```python
from build123d import *

# Parameters (mm, degrees)
SKETCH1_R           = 1
BOSS_EXTRUDE1_DEPTH = 8
SKETCH2_R           = 7
SKETCH2_R_2         = 3
CUT_EXTRUDE1_DEPTH  = 4
SKETCH3_R           = 3
CUT_EXTRUDE2_DEPTH  = 1.5
SKETCH8_R           = 3
BOSS_EXTRUDE4_DEPTH = 3
SKETCH9_W           = 12
SKETCH9_H           = 7
CUT_EXTRUDE5_DEPTH  = 19
SKETCH10_R          = 4.5
CUT_EXTRUDE11_DEPTH = 5
SKETCH12_R          = 3
CUT_EXTRUDE12_DEPTH = 5
SKETCH13_W          = 28.183943327
SKETCH13_H          = 2
CUT_EXTRUDE13_DEPTH = 19
BOSS_EXTRUDE5_REACH = 20
SKETCH14_W          = 8.331719186
SKETCH14_H          = 2


with BuildPart() as part:
    # Sketch1 → Boss-Extrude1 (new body)
    with BuildSketch(Plane(origin=(0, 0, 0), x_dir=(1, 0, 0), z_dir=(0, 1, 0))):
        with BuildLine():
            Line((-3, 53.504881109), (15, 53.504881109))
            Line((15, 53.504881109), (15, 23.504881109))
            ThreePointArc((15, 23.504881109), (6, 14.504881109), (-3, 23.504881109))
            Line((-3, 23.504881109), (-3, 53.504881109))
        make_face()
        with Locations((6, 36.504881109)):
            Circle(SKETCH1_R, mode=Mode.SUBTRACT)
        with Locations((6, 46.504881109)):
            Circle(SKETCH1_R, mode=Mode.SUBTRACT)
    extrude(amount=BOSS_EXTRUDE1_DEPTH)

    # Sketch2 → Cut-Extrude1 (cut)
    with BuildSketch(Plane(origin=(0, 8, 0), x_dir=(1, 0, 0), z_dir=(0, 1, 0))):
        with Locations((6, 23.504881109)):
            Circle(SKETCH2_R)
        with Locations((6, 23.504881109)):
            Circle(SKETCH2_R_2, mode=Mode.SUBTRACT)
    extrude(amount=-CUT_EXTRUDE1_DEPTH, mode=Mode.SUBTRACT)

    # Sketch3 → Cut-Extrude2 (cut)
    with BuildSketch(Plane(origin=(0, 8, 0), x_dir=(1, 0, 0), z_dir=(0, 1, 0))):
        with Locations((6, 23.504881109)):
            Circle(SKETCH3_R)
    extrude(amount=-CUT_EXTRUDE2_DEPTH, mode=Mode.SUBTRACT)

    # Sketch8 → Boss-Extrude4 (add)
    with BuildSketch(Plane(origin=(0, 8, 0), x_dir=(1, 0, 0), z_dir=(0, 1, 0))):
        with BuildLine():
            Line((1, 39.504881109), (11, 39.504881109))
            Line((11, 39.504881109), (15, 39.504881109))
            Line((15, 39.504881109), (15, 46.504881109))
            ThreePointArc((15, 46.504881109), (6, 51.504881109), (-3, 46.504881109))
            Line((-3, 46.504881109), (-3, 39.504881109))
            Line((-3, 39.504881109), (1, 39.504881109))
        make_face()
        with Locations((6, 46.504881109)):
            Circle(SKETCH8_R, mode=Mode.SUBTRACT)
    extrude(amount=BOSS_EXTRUDE4_DEPTH)

    # Sketch9 → Cut-Extrude5 (cut, through all)
    with BuildSketch(Plane(origin=(15, 0, 0), x_dir=(0, 0, -1), z_dir=(1, 0, 0))):
        with Locations((47.504881109, 3.5)):
            Rectangle(SKETCH9_W, SKETCH9_H)
    extrude(amount=-CUT_EXTRUDE5_DEPTH, mode=Mode.SUBTRACT)

    # Sketch10 → Cut-Extrude11 (cut)
    with BuildSketch(Plane(origin=(0, 8, 0), x_dir=(1, 0, 0), z_dir=(0, 1, 0))):
        with Locations((6, 36.504881109)):
            Circle(SKETCH10_R)
    extrude(amount=CUT_EXTRUDE11_DEPTH, mode=Mode.SUBTRACT)

    # Sketch12 → Cut-Extrude12 (cut)
    with BuildSketch(Plane(origin=(0, 8, 0), x_dir=(1, 0, 0), z_dir=(0, 1, 0))):
        with Locations((6, 46.504881109)):
            Circle(SKETCH12_R)
        with BuildLine():
            Line((-3, 53.504881109), (15, 53.504881109))
            Line((15, 53.504881109), (15, 46.504881109))
            ThreePointArc((15, 46.504881109), (6, 51.504881109), (-3, 46.504881109))
            Line((-3, 46.504881109), (-3, 53.504881109))
        make_face()
    extrude(amount=-CUT_EXTRUDE12_DEPTH, mode=Mode.SUBTRACT)

    # Sketch13 → Cut-Extrude13 (cut, through all)
    with BuildSketch(Plane(origin=(15, 0, 0), x_dir=(0, 0, -1), z_dir=(1, 0, 0))):
        with Locations((27.412909446, 1)):
            Rectangle(SKETCH13_W, SKETCH13_H)
    extrude(amount=-CUT_EXTRUDE13_DEPTH, mode=Mode.SUBTRACT)

    # Sketch14 → Boss-Extrude5 (add, up to next)
    with BuildSketch(Plane(origin=(15, 0, 0), x_dir=(0, 0, -1), z_dir=(1, 0, 0)), mode=Mode.PRIVATE) as boss_extrude5_sk1:
        with Locations((37.339021516, 3)):
            Rectangle(SKETCH14_W, SKETCH14_H)
    boss_extrude5_tool1 = extrude(boss_extrude5_sk1.sketch, amount=-BOSS_EXTRUDE5_REACH, mode=Mode.PRIVATE) - part.part
    add(boss_extrude5_tool1.solids().sort_by_distance((15, 3, -37.339022))[0])


solid = part.part
```
Design review of the part built by this model. Coordinates are the model's own, in mm. A direction names the side the tool comes from. Coordinates: 2 decimals unless noted, no trailing zeros. Order: outer loops, then holes, each group sorted by start corner. A loop starts at its lowest first (then second) coordinate and runs counter-clockwise, first axis right, second up. Notation, with made-up numbers: M 88.25,71.5 L 103.25,71.5 A12 cw 103.25,83.5 Z; hole C -28,58.5 d6. An arc over 180 degrees is marked long. Answer as a JSON object with one key per item and string values. Group by question number.
1) Add section A-A, the plane y = 5.25. Write out the cut boundary in (x, z).
2) Tool access review of faces 5 (the flat face through (0, 9, -39.505)), 6 (the cylindrical face through (5.26, 5.97, -37.18)), 7 (the flat face through (8, 7, -44)): name each direction out of +Z, -Z, +X, -X, +Y, -Y from which nothing blocks a thin tool from reaching the whole face with its end or side.
3) Mouldability with a two-part tool opening along X and no side actions: class faces 1 (the flat face through (12, 9, -39.505)), 2 (the cylindrical face through (6.198, 4.958, -14.507)), 3 (the cylindrical face through (5.089, 6.028, -30.445)), 4 (the cylindrical face through (8.771, 5.268, -22.356)) as pulls with the +X half, pulls with the -X half, needs draft (parallel to the pull), parting line crosses it, or undercut.
4) Add section D-D, the plane z = -48.5. Write out the cut boundary in (x, y), then the cut area to 3 significant figures.
5) Add section C-C, the plane y = 9.25. Write out the cut boundary in (x, z).
6) For pin 1 (8 mm diameter, centred on x = 6, z = -46.5, fed in from -Y); pin 2 (2.5 mm diameter, centred on x = 3, y = 4.5, fed in from -Z); pin 3 (1 mm diameter, centred on x = 11.5, y = 7, fed in from -Z), all flat-tipped, find the tip position at first contact; note any pin that passes through.
7) Wall thickness on L1, parallel to Z at x = 6, y = 5.8; L2, parallel to Y at x = 10, z = -47; L3, parallel to Z at x = 0.5, y = 5 (3 decimals): over which ranges is each line inside the solid? List them lowest first.
8) Add section B-B, the plane x = 6. Write out the cut boundary in (y, z).
Computed values:
{
 "1": {"outline": "M -3,-41.5 L 15,-41.5 L 15,-23.5 A9 ccw -3,-23.5 Z; C 6,-23.5 d6; hole C 6,-23.5 d14; hole C 6,-36.5 d2"},
 "2": {"face 5": "+Z, +X, -X, +Y", "face 6": "+Y", "face 7": "-Z, +X, -X, -Y"},
 "3": {"face 1": "needs draft", "face 2": "parting line crosses it", "face 3": "undercut", "face 4": "undercut"},
 "4": {"outline": "M -1.39,7 L 3.76,7 L 3.76,11 L -1.39,11 Z; M 8.24,7 L 13.39,7 L 13.39,11 L 8.24,11 Z", "area": "41.2 mm^2"},
 "5": {"outline": "M -3,-46.5 A10.6 ccw 15,-46.5 L 15,-39.5 L 9.35,-39.5 A4.5 cw 2.65,-39.5 L -3,-39.5 Z; hole C 6,-46.5 d6"},
 "6": {"pin 1": "stops at y = 7", "pin 2": "stops at z = -41.5", "pin 3": "stops at z = -50.25"},
 "7": {"L1": "z = -41.5 to -37.5, -35.5 to -30.5, -26.5 to -20.5, -16.5 to -14.5", "L2": "y = 7 to 11", "L3": "z = -41.505 to -27.835, -19.175 to -16.381"},
 "8": {"outline": "M 2,-41.5 L 7,-41.5 L 7,-43.5 L 11,-43.5 L 11,-41 L 8,-41 L 8,-37.5 L 4,-37.5 L 4,-35.5 L 8,-35.5 L 8,-30.5 L 4,-30.5 L 4,-26.5 L 6.5,-26.5 L 6.5,-20.5 L 4,-20.5 L 4,-16.5 L 8,-16.5 L 8,-14.5 L 2,-14.5 Z; M 7,-51.5 L 11,-51.5 L 11,-49.5 L 7,-49.5 Z"}
}
